from build123d import *

# Parameters (mm, degrees)
F0_W     = 50
F0_H     = 18
F1_DEPTH = 20
F2_W     = 40.5
F2_H     = 8.5
F3_DEPTH = 15
F4_SIZE  = 3


with BuildPart() as f1:
    # F0 (on Top) → F1 (new body)
    with BuildSketch(Plane.XY):
        Rectangle(F0_W, F0_H)
    extrude(amount=F1_DEPTH)

    # F2 (on face) → F3 (cut, through all)
    with BuildSketch(Plane.XY.offset(20)):
        Rectangle(F2_W, F2_H)
    extrude(amount=-F3_DEPTH, mode=Mode.SUBTRACT)

    # F4
    f4_edges = [f1.edges().sort_by_distance(p)[0] for p in [
        (0, -9, 0),
        (-25, 0, 0),
        (0, 9, 0),
        (25, 0, 0),
        (-25, -9, 10),
        (-25, 9, 10),
        (25, 9, 10),
        (25, -9, 10),
    ]]
    chamfer(f4_edges, length=F4_SIZE)


solid = f1.part
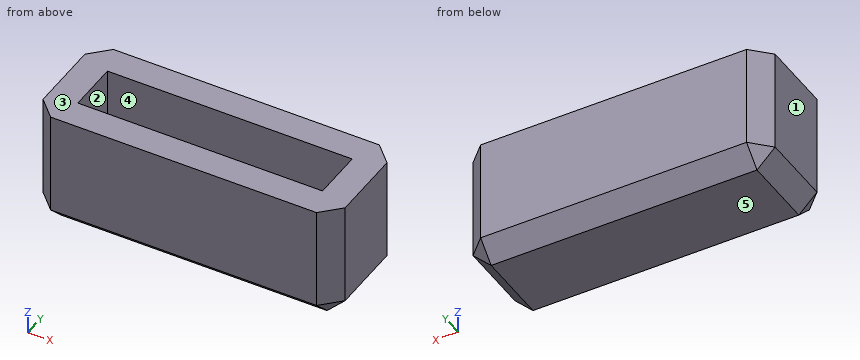
Check sheet for the modelled part. Datum: model origin and axes. Units: mm. Face numbers are marked on the shaded views. A direction names the side the tool comes from. Round coordinates to 2 decimals unless told otherwise and drop trailing zeros. Write each loop counter-clockwise with the first axis right and the second up, starting at its lowest first coordinate (ties: lowest second). Pieces come first, ordered by that corner, then holes. Notation, with made-up numbers: (35.5, 46.5) -> (58.5, 46.5) arc R23 cw to (58.5, 60.5) -> close; hole circle Ø8 at (23.5, 15.5). An arc over 180 degrees is marked (long way). Answer as CSV lines item,"result". Start each with the question number.
1) Material ranges on line 1 (X direction, y = 2.5, z = 6); line 2 (Y direction, x = 13.5, z = 5.5); line 3 (Z direction, x = 20, y = 1.25), recorded low to high. Write a range as from..to.
2) Section check B-B on x = 17.5. Enter the section's corners in (y, z), and give its area (4 significant figures).
3) Section check D-D on z = 3.5. Enter the section's corners in (x, y).
4) Release check for a two-part mould opening along X. For the marked faces 1, 2 and 3 record: pulls with the +X half, pulls with the -X half, needs draft (parallel to the pull), parting line crosses it, or undercut.
5) Tool access check on the marked faces 4 and 5. Record the directions out of +Z, -Z, +X, -X, +Y, -Y that give a thin tool (end or side, any length) a straight path to the whole face; none if there is none.
6) Section check C-C on y = 2.5. Enter the section's corners in (x, z), and give its area (4 significant figures).
7) Section check A-A on z = 18.5. Enter the section's corners in (x, y), and give its area (3 significant figures).
Found:
1,line 1,"x = -25..-20.25, 20.25..25"
1,line 2,"y = -9..-4.25, 4.25..9"
1,line 3,"z = 0..5"
2,outline,"(-9, 3) -> (-6, 0) -> (6, 0) -> (9, 3) -> (9, 20) -> (4.25, 20) -> (4.25, 5) -> (-4.25, 5) -> (-4.25, 20) -> (-9, 20) -> close"
2,area,"223.5 mm^2"
3,outline,"(-25, -6) -> (-22, -9) -> (22, -9) -> (25, -6) -> (25, 6) -> (22, 9) -> (-22, 9) -> (-25, 6) -> close"
4,face 1,"pulls with the -X half"
4,face 2,"undercut"
4,face 3,"needs draft"
5,face 4,"+Z"
5,face 5,"-Z, +X, -X, +Y, -Y"
6,outline,"(-25, 3) -> (-22, 0) -> (22, 0) -> (25, 3) -> (25, 20) -> (20.25, 20) -> (20.25, 5) -> (-20.25, 5) -> (-20.25, 20) -> (-25, 20) -> close"
6,area,"383.5 mm^2"
7,outline,"(-25, -6) -> (-22, -9) -> (22, -9) -> (25, -6) -> (25, 6) -> (22, 9) -> (-22, 9) -> (-25, 6) -> close; hole (-20.25, -4.25) -> (20.25, -4.25) -> (20.25, 4.25) -> (-20.25, 4.25) -> close"
7,area,"538 mm^2"
